from build123d import *

# Parameters (mm, degrees)
BOSS_EXTRUDE2_DEPTH     = 30
SKETCH2_R               = 31
BOSS_EXTRUDE3_DEPTH     = 5
FILLET1_R               = 1
BOSS_EXTRUDE4_START     = 5.5
SKETCH3_R               = 31
SKETCH3_R_2             = 11
BOSS_EXTRUDE4_DEPTH     = 5.5
CUT_EXTRUDE1_DEPTH      = 51.222007128
CUT_EXTRUDE1_DEPTH_BACK = 51.222007128
SKETCH4_R               = 2
CUT_EXTRUDE2_DEPTH      = 54.122499941
CUT_EXTRUDE2_DEPTH_BACK = 54.122499941
SKETCH6_R               = 2.5
FILLET2_R               = 1


with BuildPart() as part:
    # Sketch1 → Boss-Extrude2 (new body)
    with BuildSketch(Plane(origin=(0, 0, 0), x_dir=(1, 0, 0), z_dir=(0, 1, 0))):
        with BuildLine():
            Line((0, 5.5), (0, 3))
            ThreePointArc((0, 3), (-3, 0), (0, -3))
            Line((0, -3), (0, -5.5))
            ThreePointArc((0, -5.5), (-5.5, 0), (0, 5.5))
        make_face()
    extrude(amount=BOSS_EXTRUDE2_DEPTH)

    # Sketch2 → Boss-Extrude3 (add)
    with BuildSketch(Plane(origin=(0, 0, 0), x_dir=(1, 0, 0), z_dir=(0, 1, 0))):
        with Locations(Location((0, 0, 0), (0, 0, 270))):
            Circle(SKETCH2_R)
    extrude(amount=-BOSS_EXTRUDE3_DEPTH)

    # Fillet1
    fillet1_edges = [part.edges().sort_by_distance(p)[0] for p in [
        (-5.5, 0, 0),
    ]]
    fillet(fillet1_edges, radius=FILLET1_R)

    # Sketch3 → Boss-Extrude4 (add)
    with BuildSketch(Plane(origin=(0, 0, 0), x_dir=(1, 0, 0), z_dir=(0, 1, 0)).offset(BOSS_EXTRUDE4_START)):
        with Locations(Location((0, 0, 0), (0, 0, 270))):
            Circle(SKETCH3_R)
        with Locations(Location((0, 0, 0), (0, 0, 270))):
            Circle(SKETCH3_R_2, mode=Mode.SUBTRACT)
    extrude(amount=-BOSS_EXTRUDE4_DEPTH)

    # Sketch4 → Cut-Extrude1 (cut, two sides: drawn at the far end of the back side and taken through both)
    with BuildSketch(Plane(origin=(0, 5.5, 0), x_dir=(1, 0, 0), z_dir=(0, 1, 0)).offset(-CUT_EXTRUDE1_DEPTH_BACK)):
        with Locations(Location((0, 21, 0), (0, 0, 270))):
            Circle(SKETCH4_R)
        with Locations(Location((21.125, -0.125, 0), (0, 0, 270))):
            Circle(SKETCH4_R)
        with Locations(Location((0, -21.25, 0), (0, 0, 270))):
            Circle(SKETCH4_R)
        with Locations(Location((-21.125, -0.125, 0), (0, 0, 270))):
            Circle(SKETCH4_R)
    extrude(amount=CUT_EXTRUDE1_DEPTH + CUT_EXTRUDE1_DEPTH_BACK, mode=Mode.SUBTRACT)

    # Sketch6 → Cut-Extrude2 (cut, two sides: drawn at the far end of the back side and taken through both)
    with BuildSketch(Plane(origin=(0, 0, 0), x_dir=(0, 0, -1), z_dir=(1, 0, 0)).offset(-CUT_EXTRUDE2_DEPTH_BACK)):
        with Locations((0, 11)):
            Circle(SKETCH6_R)
    extrude(amount=CUT_EXTRUDE2_DEPTH + CUT_EXTRUDE2_DEPTH_BACK, mode=Mode.SUBTRACT)

    # Fillet2
    fillet2_edges = [part.edges().sort_by_distance(p)[0] for p in [
        (-3, 0, 0),
    ]]
    fillet(fillet2_edges, radius=FILLET2_R)


solid = part.part
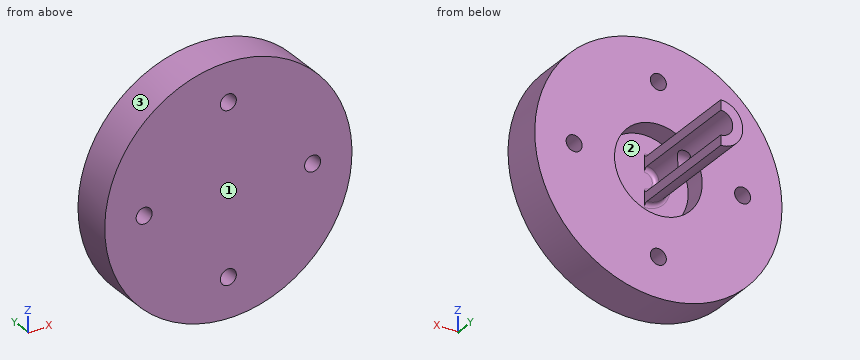
Input: part model. Units: mm. Frame: model coordinates. Face numbers are marked on the shaded views. Give positions to 0.01 mm unless a question says otherwise; leave off trailing zeros. Write each loop counter-clockwise with the first axis right and the second up, starting at its lowest first coordinate (ties: lowest second). Pieces come first, ordered by that corner, then holes.
Q1. Section C-C, the plane y = 12. Output: boundary loops of the cut face in (x, z).
Q2. First-contact query: P1, Ø2, axis at x = 23, z = 10, coming from the +Y side; P2, Ø12, axis at y = 26.5, z = 10, coming from the +X side. Flat tips, straight axial feed; report the tip coordinate or a pass-through.
Q3. Section A-A, the plane y = 3. Output: boundary loops of the cut face in (x, z) (3 decimals).
Q4. Pull-direction query (X, two-part tool) for the marked faces 1, 2 and 3; classes: pulls with the +X half, pulls with the -X half, needs draft (parallel to the pull), parting line crosses it, or undercut.
Q5. Section D-D, the plane z = 21.25. Output: boundary loops of the cut face in (x, y).
Q6. Section B-B, the plane z = 0. Output: boundary loops of the cut face in (x, y), plus the area to 3 significant figures.
Q7. Material intervals for probe 1 along X at (y, z) = (1.6, 0); probe 2 along Y at (x, z) = (-15.5, -18); probe 3 along X at (y, z) = (-1.25, -21), sorted ascending.
Filled in:
1. outline: (-5, -2.29) arc R5.5 ccw to (0, -5.5) - (0, -3) arc R3 cw to (-1.94, -2.29) - close; (-5, 2.29) - (-1.94, 2.29) arc R3 cw to (0, 3) - (0, 5.5) arc R5.5 ccw to start
2. P1: stops at y = 5.5
2. P2: stops at x = 0
3. outline: circle Ø62 at (0, 0); (0, -5.5) - (0, -3) arc R3 cw to (0, 3) - (0, 5.5) arc R5.5 ccw to start; hole circle Ø4 at (-21.125, 0.125); hole circle Ø22 at (0, 0); hole circle Ø4 at (0, -21); hole circle Ø4 at (0, 21.25); hole circle Ø4 at (21.125, 0.125)
4. face 1: needs draft
4. face 2: undercut
4. face 3: parting line crosses it
5. outline: (-22.57, -5) - (-2, -5) - (-2, 5.5) - (-22.57, 5.5) - close; (2, -5) - (22.57, -5) - (22.57, 5.5) - (2, 5.5) - close
6. outline: (-31, -5) - (-23.12, -5) - (-23.12, 5.5) - (-31, 5.5) - close; (-19.13, -5) - (19.13, -5) - (19.13, 5.5) - (11, 5.5) - (11, 0) - (-2, 0) arc R1 cw to (-3, 1) - (-3, 8.5) - (-5.5, 8.5) - (-5.5, 1) arc R1 cw to (-6.5, 0) - (-11, 0) - (-11, 5.5) - (-19.13, 5.5) - close; (-5.5, 13.5) - (-3, 13.5) - (-3, 30) - (-5.5, 30) - close; (23.12, -5) - (31, -5) - (31, 5.5) - (23.12, 5.5) - close
6. area: 509 mm2
7. probe 1: x = -31 to -23.12, -19.13 to -11, -5.5 to -3, 11 to 19.13, 23.12 to 31
7. probe 2: y = -5 to 5.5
7. probe 3: x = -22.8 to -2, 2 to 22.8
